from build123d import *

# Parameters (mm, degrees)
SKETCH_1_R               = 55
EXTRUDE_1_DEPTH          = 3
PATTERN_CIRCULAR_1_COUNT = 6
SKETCH_5_R               = 17.5
CUT_EXTRUDE_1_DEPTH      = 1
CHAMFER_1_SIZE           = 1


with BuildPart() as part:
    # 草图1 → 凸台-拉伸1 (new body)
    with BuildSketch(Plane(origin=(0, 0, 0), x_dir=(1, 0, 0), z_dir=(0, 1, 0))):
        with Locations(Location((0, 0, 0), (0, 0, 270))):
            Circle(SKETCH_1_R)
    extrude(amount=EXTRUDE_1_DEPTH)

    # 草图4 → M8 螺纹孔的螺纹孔钻头1 (revolve, cut)
    with BuildSketch(Plane(origin=(0, 3, -45), x_dir=(0, 0, 1), z_dir=(1, 0, 0))):
        Polygon((0, 0), (0, 18.042926105), (3.4, 16), (3.4, 0), align=None)
    hole_wizard_m8_1 = revolve(axis=Axis((0, 9.35, -45), (0, -1, 0)), mode=Mode.SUBTRACT)

    # 阵列(圆周)1: M8 螺纹孔的螺纹孔钻头1 ×6 about axis
    pattern_circular_1_axis = Axis((0, 0, 0), (0, 1, 0))
    for i in range(1, PATTERN_CIRCULAR_1_COUNT):
        add(hole_wizard_m8_1.rotate(pattern_circular_1_axis, i * 360 / PATTERN_CIRCULAR_1_COUNT), mode=Mode.SUBTRACT)

    # 草图5 → 切除-拉伸1 (cut)
    with BuildSketch(Plane(origin=(0, 3, 0), x_dir=(1, 0, 0), z_dir=(0, 1, 0))):
        with Locations(Location((0, 0, 0), (0, 0, 270))):
            Circle(SKETCH_5_R)
    extrude(amount=-CUT_EXTRUDE_1_DEPTH, mode=Mode.SUBTRACT)

    # 倒角1
    chamfer_1_edges = [part.edges().sort_by_distance(p)[0] for p in [
        (0, 0, -55),
        (0, 3, -17.5),
        (0, 3, -55),
    ]]
    chamfer(chamfer_1_edges, length=CHAMFER_1_SIZE - 0.0001)  # a hair under: the kernel refuses the full size


solid = part.part
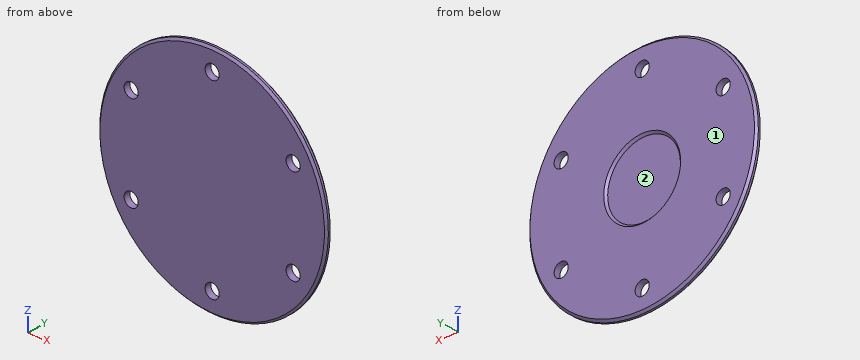
Here's how the part is built. I have some questions about the finished solid (model axes, mm). Face numbers are marked on the shaded views. Coordinates: 2 decimals unless noted, no trailing zeros. Write each loop counter-clockwise with the first axis right and the second up, starting at its lowest first coordinate (ties: lowest second). Pieces come first, ordered by that corner, then holes.
1) If we section it at B-B (y = 1.55): List the corners of the cut face in (x, z) for me, plus the area to 3 significant figures.
Filled in:
outline: circle Ø110 at (0, 0); hole circle Ø6.8 at (-38.97, -22.5); hole circle Ø6.8 at (-38.97, 22.5); hole circle Ø6.8 at (0, -45); hole circle Ø6.8 at (0, 45); hole circle Ø6.8 at (38.97, -22.5); hole circle Ø6.8 at (38.97, 22.5)
area: 9,290 mm2
2) Thinking about a two-plate mould opening in X: for the marked faces 1 and 2, which applies, +X half, -X half, draft (parallel to the pull), parting line (faces both ways), or undercut?
Filled in:
face 1: draft
face 2: undercut
3) If we section it at A-A (x = 0): Count the separate pieces of the cut face and the enclosed holes in it, plus the area to 3 significant figures.
Filled in:
separate pieces: 3
enclosed holes: 0
area: 251 mm2
4) If I drill on line 1 (Z direction, x = -40, y = 0.85); line 2 (Z direction, x = -40, y = 2.6); line 3 (X direction, y = 2.05, z = 22.5), over which ranges is the centre line in solid material (lowest first)?
Filled in:
line 1: z = -37.53 to -25.74, -19.26 to 19.26, 25.74 to 37.53
line 2: z = -36.87 to -25.74, -19.26 to 19.26, 25.74 to 36.87
line 3: x = -50.13 to -42.37, -35.57 to 35.57, 42.37 to 50.13
5) I'm going to push a flat-ended pin straight in: pin 1 (17.5 mm diameter, centred on x = -3, z = -3, fed in from +Y). Where does the tip first touch, or does it pass through?
Filled in:
pin 1: stops at y = 2
